Geometry check sheet. Reference: the model listing, model coordinates, mm. A direction names the side the tool comes from. Round coordinates to 2 decimals unless told otherwise and drop trailing zeros. Loops run counter-clockwise (first coordinate to the right, second up) from the corner with the lowest first, then second, coordinate; pieces in that order, holes last. Notation, with made-up numbers: (83.5, 65) - (119.5, 65) arc R29 cw to (119.5, 97) - close; hole circle Ø4 at (19.5, 76). An arc over 180 degrees is marked (long way). Write item = value, one per line.
```python
from build123d import *

# Parameters (mm, degrees)
SKETCH_1_W          = 72
SKETCH_1_H          = 16
EXTRUDE_1_DEPTH     = 1.2
FILLET_1_R          = 3
CUT_EXTRUDE_1_REACH = 75.766
SKETCH_3_R          = 1.2
CUT_EXTRUDE_2_REACH = 75.766
SKETCH_4_W          = 9
SKETCH_4_H          = 6
FILLET_2_R          = 1


with BuildPart() as part:
    # 草图1 → 凸台-拉伸1 (new body)
    with BuildSketch(Plane.XY):
        with Locations((36, 8)):
            Rectangle(SKETCH_1_W, SKETCH_1_H)
    extrude(amount=EXTRUDE_1_DEPTH)

    # 圆角1
    fillet_1_edges = [part.edges().sort_by_distance(p)[0] for p in [
        (0, 16, 0.6),
        (72, 16, 0.6),
        (72, 0, 0.6),
        (0, 0, 0.6),
    ]]
    fillet(fillet_1_edges, radius=FILLET_1_R)

    # 草图3 → 切除-拉伸1 (cut, up to next)
    with BuildSketch(Plane(origin=(0, 0, 0), x_dir=(-1, 0, 0), z_dir=(0, 0, -1)), mode=Mode.PRIVATE) as cut_extrude_1_sk1:
        with Locations((-70.012877826, 14.013032766)):
            Circle(SKETCH_3_R)
    cut_extrude_1_tool1 = extrude(cut_extrude_1_sk1.sketch, amount=-CUT_EXTRUDE_1_REACH, mode=Mode.PRIVATE) & part.part
    # 草图3 → 切除-拉伸1 (cut, up to next)
    with BuildSketch(Plane(origin=(0, 0, 0), x_dir=(-1, 0, 0), z_dir=(0, 0, -1)), mode=Mode.PRIVATE) as cut_extrude_1_sk2:
        with Locations((-70.012694945, 2.012672085)):
            Circle(SKETCH_3_R)
    cut_extrude_1_tool2 = extrude(cut_extrude_1_sk2.sketch, amount=-CUT_EXTRUDE_1_REACH, mode=Mode.PRIVATE) & part.part
    # 草图3 → 切除-拉伸1 (cut, up to next)
    with BuildSketch(Plane(origin=(0, 0, 0), x_dir=(-1, 0, 0), z_dir=(0, 0, -1)), mode=Mode.PRIVATE) as cut_extrude_1_sk3:
        with Locations((-2.011949988, 14.012003328)):
            Circle(SKETCH_3_R)
    cut_extrude_1_tool3 = extrude(cut_extrude_1_sk3.sketch, amount=-CUT_EXTRUDE_1_REACH, mode=Mode.PRIVATE) & part.part
    # 草图3 → 切除-拉伸1 (cut, up to next)
    with BuildSketch(Plane(origin=(0, 0, 0), x_dir=(-1, 0, 0), z_dir=(0, 0, -1)), mode=Mode.PRIVATE) as cut_extrude_1_sk4:
        with Locations((-2.012501905, 2.013009906)):
            Circle(SKETCH_3_R)
    cut_extrude_1_tool4 = extrude(cut_extrude_1_sk4.sketch, amount=-CUT_EXTRUDE_1_REACH, mode=Mode.PRIVATE) & part.part
    add(cut_extrude_1_tool1.solids().sort_by_distance((70.012878, 14.013033, 0))[0], mode=Mode.SUBTRACT)
    add(cut_extrude_1_tool2.solids().sort_by_distance((70.012695, 2.012672, 0))[0], mode=Mode.SUBTRACT)
    add(cut_extrude_1_tool3.solids().sort_by_distance((2.01195, 14.012003, 0))[0], mode=Mode.SUBTRACT)
    add(cut_extrude_1_tool4.solids().sort_by_distance((2.012502, 2.01301, 0))[0], mode=Mode.SUBTRACT)

    # 草图4 → 切除-拉伸2 (cut, up to next)
    with BuildSketch(Plane(origin=(0, 0, 0), x_dir=(-1, 0, 0), z_dir=(0, 0, -1)), mode=Mode.PRIVATE) as cut_extrude_2_sk1:
        with Locations((-51.5, 13.4)):
            Rectangle(SKETCH_4_W, SKETCH_4_H)
    cut_extrude_2_tool1 = extrude(cut_extrude_2_sk1.sketch, amount=-CUT_EXTRUDE_2_REACH, mode=Mode.PRIVATE) & part.part
    add(cut_extrude_2_tool1.solids().sort_by_distance((51.5, 13.4, 0))[0], mode=Mode.SUBTRACT)

    # 圆角2
    fillet_2_edges = [part.edges().sort_by_distance(p)[0] for p in [
        (56, 16, 0.6),
        (47, 16, 0.6),
        (56, 10.4, 0.6),
        (47, 10.4, 0.6),
    ]]
    fillet(fillet_2_edges, radius=FILLET_2_R)


solid = part.part
```
(1) Mould release check, pull along X, two halves, no side actions. Record for faces 3 (the flat face through (72, 8, 1)), 4 (the flat face through (56, 13, 1)), 5 (the cylindrical face through (0.86, 0.9, 0.61)): pulls with the +X half, pulls with the -X half, needs draft (parallel to the pull), parting line crosses it, or undercut.
Answers follow:
face_3 = pulls with the +X half
face_4 = undercut
face_5 = pulls with the -X half
(2) Gauge pin test, flat end, axial feed: pin 1 (0.6 mm diameter, centred on x = 53, z = 0.5, fed in from +Y). Record the tip position at first contact, or that the pin passes through.
Answers follow:
pin_1 = 10.4
(3) Scan lines: L1, parallel to X at y = 15, z = 0.6; L2, parallel to X at y = 11.5, z = 0.25; L3, parallel to X at y = 1.25, z = 0.95. Record each from-to range of solid material in increasing order. Write a range as [from, to].
Answers follow:
L1 = [0.76, 1.33], [2.69, 47], [56, 69.33], [70.7, 71.24]
L2 = [0, 47], [56, 72]
L3 = [0.56, 1.09], [2.94, 69.09], [70.94, 71.44]
(4) Set-up check for faces 1 (the flat face through (47, 13, 1)), 2 (the flat face through (35, 8, 0)): record each of +Z, -Z, +X, -X, +Y, -Y from which the full face is reachable in a straight line by a thin tool's end or side.
Answers follow:
face_1 = +Z, -Z, +Y
face_2 = -Z, +X, -X, +Y, -Y
(5) Section check A-A (z = 0.25). Enter the section's corners in (x, y), then the cut area to 3 significant figures.
Answers follow:
outline = (0, 3) arc R3 ccw to (3, 0) - (69, 0) arc R3 ccw to (72, 3) - (72, 13) arc R3 ccw to (69, 16) - (57, 16) arc R1 ccw to (56, 15) - (56, 11.4) arc R1 cw to (55, 10.4) - (48, 10.4) arc R1 cw to (47, 11.4) - (47, 15) arc R1 ccw to (46, 16) - (3, 16) arc R3 ccw to (0, 13) - close; hole circle Ø2.4 at (2.01, 2.01); hole circle Ø2.4 at (2.01, 14.01); hole circle Ø2.4 at (70.01, 2.01); hole circle Ø2.4 at (70.01, 14.01)
area = 1,080 mm²
